Geometry check sheet. Reference: the model listing, model coordinates, mm. Face numbers are marked on the shaded views. A direction names the side the tool comes from. Coordinates: 2 decimals unless noted, no trailing zeros. Write each loop counter-clockwise with the first axis right and the second up, starting at its lowest first coordinate (ties: lowest second). Pieces come first, ordered by that corner, then holes. Notation, with made-up numbers: (34.25, 31) -> (80.25, 31) arc R32 ccw to (80.25, 68) -> close; hole circle Ø1 at (-32.75, 60). An arc over 180 degrees is marked (long way). Answer in a Markdown table with one row per item. Add a question column.
Q1. Tool access check on the marked faces 5 and 6. Record the directions out of +Z, -Z, +X, -X, +Y, -Y that give a thin tool (end or side, any length) a straight path to the whole face; none if there is none.
Q2. Section check B-B, the plane z = 2.5. Record the boundary of the cut face in (x, y).
Q3. Section check C-C, the plane x = -4. Record the boundary of the cut face in (y, z).
Q4. Section check D-D, the plane z = 17. Record the boundary of the cut face in (x, y).
Q5. Section check A-A, the plane y = -12. Record the boundary of the cut face in (x, z), and give its area (3 significant figures).
Q6. Thickness scan on line 1 (X direction, y = 0.25, z = 20.25); line 2 (Z direction, x = -12, y = 6); line 3 (Z direction, x = 18, y = -13.25). Record the ranges inside material, lowest first.
Q7. Gauge pin test, flat ends, axial feed: P1, Ø12.5, axis at x = -11, y = -5, coming from the +Z side; P2, Ø6, axis at x = -15, z = 4, coming from the -Y side; P3, Ø7.5, axis at y = 6, z = 24, coming from the -X side. Record the tip position at first contact, or that the pin passes through.
Q8. Release check for a two-part mould opening along X. For the marked faces 1, 2, 3 and 4 record: pulls with the +X half, pulls with the -X half, needs draft (parallel to the pull), parting line crosses it, or undercut.
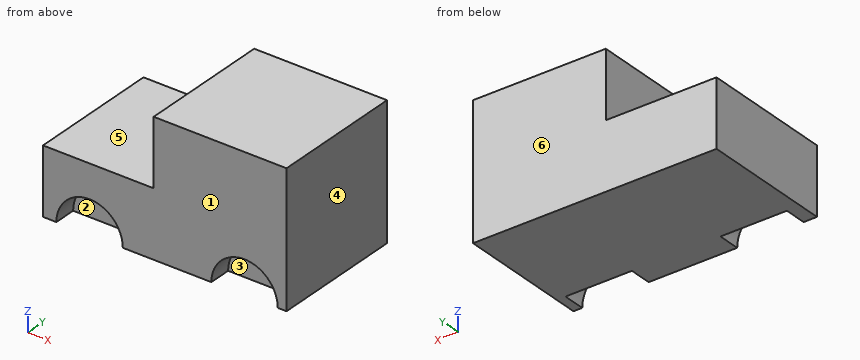
```python
from build123d import *

# Parameters (mm, degrees)
F0_W     = 55
F0_H     = 30
F1_DEPTH = 30
F2_W     = 25
F2_H     = 15
F3_DEPTH = 30.001
F5_DEPTH = 5


with BuildPart() as f1:
    # F0 (on Top) → F1 (new body)
    with BuildSketch(Plane.XY):
        Rectangle(F0_W, F0_H)
    extrude(amount=F1_DEPTH)

    # F2 (on face) → F3 (cut, through all)
    with BuildSketch(Plane.XZ.offset(15)):
        with Locations((-15, 22.5)):
            Rectangle(F2_W, F2_H)
    extrude(amount=-F3_DEPTH, mode=Mode.SUBTRACT)

    # F4 (on face) → F5 (cut)
    with BuildSketch(Plane.XZ.offset(15)):
        with BuildLine():
            Line((-24.4766619802, 0), (-9.4766619802, 0))
            ThreePointArc((-9.4766619802, 0), (-16.9766619802, 7.5), (-24.4766619802, 0))
        make_face()
        with BuildLine():
            ThreePointArc((25.5233380198, 0), (18.0233380198, 7.5), (10.5233380198, 0))
            Line((10.5233380198, 0), (25.5233380198, 0))
        make_face()
    extrude(amount=-F5_DEPTH, mode=Mode.SUBTRACT)


solid = f1.part
```
Calculated:
| question | item | result |
|---|---|---|
| 1 | face 5 | +Z, -X, +Y, -Y |
| 1 | face 6 | +Z, -Z, +X, -X, +Y |
| 2 | outline | (-27.5, -15) -> (-24.05, -15) -> (-24.05, -10) -> (-9.91, -10) -> (-9.91, -15) -> (10.95, -15) -> (10.95, -10) -> (25.09, -10) -> (25.09, -15) -> (27.5, -15) -> (27.5, 15) -> (-27.5, 15) -> close |
| 3 | outline | (-15, 0) -> (15, 0) -> (15, 15) -> (-15, 15) -> close |
| 4 | outline | (-2.5, -15) -> (27.5, -15) -> (27.5, 15) -> (-2.5, 15) -> close |
| 5 | outline | (-27.5, 0) -> (-24.48, 0) arc R7.5 cw to (-9.48, 0) -> (10.52, 0) arc R7.5 cw to (25.52, 0) -> (27.5, 0) -> (27.5, 30) -> (-2.5, 30) -> (-2.5, 15) -> (-27.5, 15) -> close |
| 5 | area | 1,100 mm² |
| 6 | line 1 | x = -2.5 to 27.5 |
| 6 | line 2 | z = 0 to 15 |
| 6 | line 3 | z = 7.5 to 30 |
| 7 | P1 | stops at z = 15 |
| 7 | P2 | stops at y = -10 |
| 7 | P3 | stops at x = -2.5 |
| 8 | face 1 | needs draft |
| 8 | face 2 | undercut |
| 8 | face 3 | undercut |
| 8 | face 4 | pulls with the +X half |
